For this review, use the dimensioned drawing (mm, ordinates from the lowest corner) and the shaded views. Round coordinates to 2 decimals unless told otherwise and drop trailing zeros. Order: outer loops, then holes, each group sorted by start corner. A loop starts at its lowest first (then second) coordinate and runs counter-clockwise, first axis right, second up. Notation, with made-up numbers: (-6.75, -34.5) - (3.25, -34.5) arc R22 cw to (3.25, -22.5) - close; hole circle Ø9 at (-18.75, 70.25). An arc over 180 degrees is marked (long way). Write item = value, one per line.
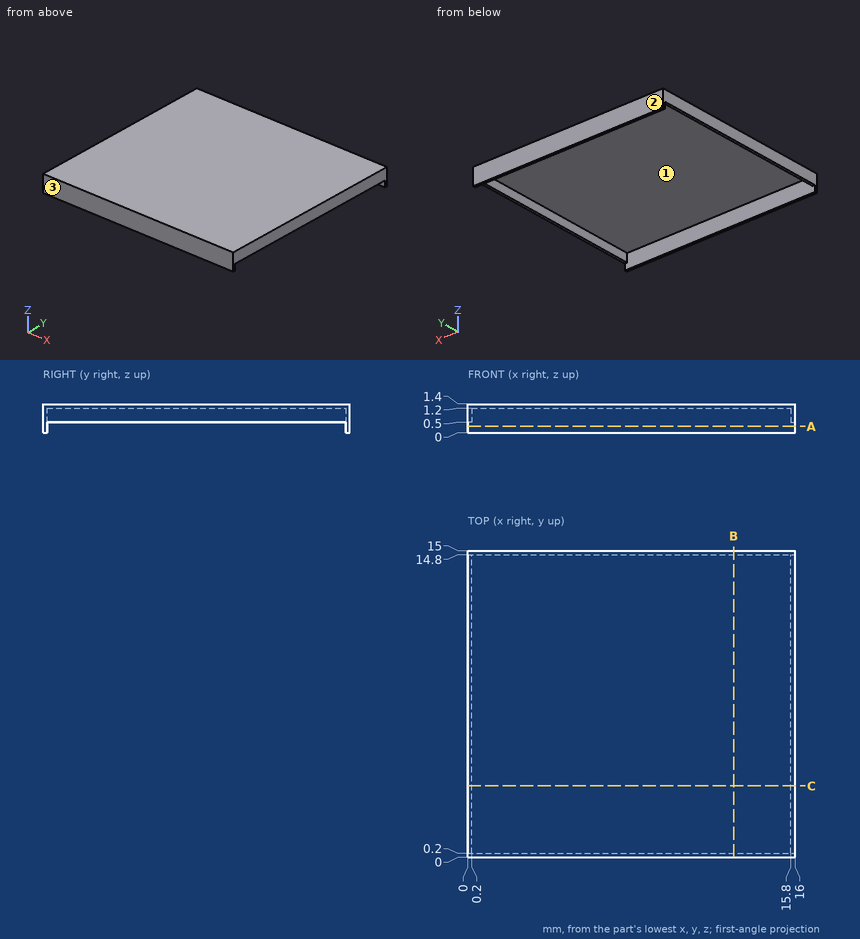
Item 1: Take a section at C-C, the plane y = 3.5. State the section outline as (x, z) points.
Data:
outline = (0, 0.5) - (0.2, 0.5) - (0.2, 1.2) - (15.8, 1.2) - (15.8, 0.5) - (16, 0.5) - (16, 1.4) - (0, 1.4) - close
Item 2: Take a section at A-A, the plane z = 0.3. State the section outline as (x, y) points, and give its area (3 significant figures).
Data:
outline = (0, 0) - (16, 0) - (16, 0.2) - (0, 0.2) - close; (0, 14.8) - (16, 14.8) - (16, 15) - (0, 15) - close
area = 6.40 mm2
Item 3: Take a section at B-B, the plane x = 13. State the section outline as (y, z) points.
Data:
outline = (0, 0) - (0.2, 0) - (0.2, 1.2) - (14.8, 1.2) - (14.8, 0) - (15, 0) - (15, 1.4) - (0, 1.4) - close
Item 4: The part is to be moulded in two halves that separate along Y. For the marked faces 1, 2 and 3, say which applies: +Y half, -Y half, draft (parallel to the pull), parting line (faces both ways), or undercut.
Data:
face_1 = undercut
face_2 = +Y half
face_3 = -Y half
Item 5: For line 1 along Y through (x, z) = (7.5, 0.5); line 2 along X through (y, z) = (4.5, 0.6); line 3 along Z through (x, y) = (11.75, 9), list the stretches that pass through material, from the lowest coordinate up. Write a range as [from, to].
Data:
line_1 = [0, 0.2], [14.8, 15]
line_2 = [0, 0.2], [15.8, 16]
line_3 = [1.2, 1.4]
